from build123d import *

# Parameters (mm, degrees)
ESQUISSE1_W                          = 61
ESQUISSE1_H                          = 41
BOSS_EXTRU_1_DEPTH                   = 100
ENL_V_MAT_EXTRU_1_DEPTH              = 57
ESQUISSE6_W                          = 58
ESQUISSE6_H                          = 3
BOSS_EXTRU_2_DEPTH                   = 4
ESQUISSE7_W                          = 35
ESQUISSE7_H                          = 3
BOSS_EXTRU_3_DEPTH                   = 6
ESQUISSE11_W                         = 58
ESQUISSE11_H                         = 3
BOSS_EXTRU_4_DEPTH                   = 7
ESQUISSE12_W                         = 59.546555331
ESQUISSE12_H                         = 3
BOSS_EXTRU_5_DEPTH                   = 5
R_P_TITION_LIN_AIRE1_COUNT           = 2
R_P_TITION_LIN_AIRE1_PITCH           = 13
R_P_TITION_LIN_AIRE1_COPY_1_SKETCH_W = 59.546555331
R_P_TITION_LIN_AIRE1_COPY_1_SKETCH_H = 3
R_P_TITION_LIN_AIRE1_COPY_1_DEPTH    = 5
ESQUISSE13_W                         = 15
ESQUISSE13_H                         = 3
BOSS_EXTRU_6_DEPTH                   = 5
R_P_TITION_LIN_AIRE3_COUNT           = 2
R_P_TITION_LIN_AIRE3_PITCH           = 4
ESQUISSE14_W                         = 15
ESQUISSE14_H                         = 7
BOSS_EXTRU_7_DEPTH                   = 16
ESQUISSE15_W                         = 2
ESQUISSE15_H                         = 1
ENL_V_MAT_EXTRU_2_DEPTH              = 14
ENL_V_MAT_EXTRU_3_DEPTH              = 15
ESQUISSE17_W                         = 59.954419869
ESQUISSE17_H                         = 3
BOSS_EXTRU_8_DEPTH                   = 15
ESQUISSE18_W                         = 20.5
ESQUISSE18_H                         = 21
ENL_V_MAT_EXTRU_4_DEPTH              = 62


with BuildPart() as part:
    # Esquisse1 → Boss.-Extru.1 (new body)
    with BuildSketch(Plane(origin=(0, 0, 0), x_dir=(1, 0, 0), z_dir=(0, 1, 0))):
        Rectangle(ESQUISSE1_W, ESQUISSE1_H)
    extrude(amount=BOSS_EXTRU_1_DEPTH)

    # Esquisse3 → Enlèv. mat.-Extru.1 (cut)
    with BuildSketch(Plane(origin=(30.5, 0, 0), x_dir=(0, 0, -1), z_dir=(1, 0, 0))):
        Polygon((17.5, 13), (17.5, 97), (-17.5, 97), (-17.5, 3), (14, 3), (14, 13), align=None)
    extrude(amount=-ENL_V_MAT_EXTRU_1_DEPTH, mode=Mode.SUBTRACT)

    # Esquisse6 → Boss.-Extru.2 (add)
    with BuildSketch(Plane(origin=(0, 0, -20.5), x_dir=(-1, 0, 0), z_dir=(0, 0, -1))):
        with Locations((-1.5, 11.5)):
            Rectangle(ESQUISSE6_W, ESQUISSE6_H)
    boss_extru_2 = extrude(amount=-BOSS_EXTRU_2_DEPTH)

    # Symétrie1: Boss.-Extru.2 across plane
    add(boss_extru_2.mirror(Plane.XY))

    # Esquisse7 → Boss.-Extru.3 (add)
    with BuildSketch(Plane.ZY.offset(30.5)):
        with Locations((0, 11.5)):
            Rectangle(ESQUISSE7_W, ESQUISSE7_H)
    extrude(amount=-BOSS_EXTRU_3_DEPTH)

    # Esquisse11 → Boss.-Extru.4 (add)
    with BuildSketch(Plane(origin=(0, 0, -20.5), x_dir=(-1, 0, 0), z_dir=(0, 0, -1))):
        with Locations((-1.5, 11.5)):
            Rectangle(ESQUISSE11_W, ESQUISSE11_H)
    extrude(amount=-BOSS_EXTRU_4_DEPTH)

    # Esquisse12 → Boss.-Extru.5 (add)
    with BuildSketch(Plane(origin=(0, 0, -20.5), x_dir=(-1, 0, 0), z_dir=(0, 0, -1))):
        with Locations((-0.726722335, 51.5)):
            Rectangle(ESQUISSE12_W, ESQUISSE12_H)
    boss_extru_5 = extrude(amount=-BOSS_EXTRU_5_DEPTH)

    # Symétrie2: Boss.-Extru.5 across plane
    add(boss_extru_5.mirror(Plane.XY))

    # Répétition linéaire1: Boss.-Extru.5 ×2
    with Locations(*[(0, -i * R_P_TITION_LIN_AIRE1_PITCH, 0) for i in range(1, R_P_TITION_LIN_AIRE1_COUNT)]):
        add(boss_extru_5)

    # Répétition linéaire1 copy 1 sketch → Répétition linéaire1 copy 1 (add)
    with BuildSketch(Plane(origin=(0, -13, 20.5), x_dir=(-1, 0, 0), z_dir=(0, 0, 1))):
        with Locations((-0.726722335, -51.5)):
            Rectangle(R_P_TITION_LIN_AIRE1_COPY_1_SKETCH_W, R_P_TITION_LIN_AIRE1_COPY_1_SKETCH_H)
    extrude(amount=-R_P_TITION_LIN_AIRE1_COPY_1_DEPTH)

    # Esquisse13 → Boss.-Extru.6 (add)
    with BuildSketch(Plane.XY.offset(20.5)):
        with Locations((-20, 81.5)):
            Rectangle(ESQUISSE13_W, ESQUISSE13_H)
    boss_extru_6 = extrude(amount=-BOSS_EXTRU_6_DEPTH)

    # Répétition linéaire3: Boss.-Extru.6 ×2
    with Locations(*[(0, i * R_P_TITION_LIN_AIRE3_PITCH, 0) for i in range(1, R_P_TITION_LIN_AIRE3_COUNT)]):
        add(boss_extru_6)

    # Esquisse14 → Boss.-Extru.7 (add)
    with BuildSketch(Plane(origin=(0, 0, -20.5), x_dir=(-1, 0, 0), z_dir=(0, 0, -1))):
        with Locations((20, 83.5)):
            Rectangle(ESQUISSE14_W, ESQUISSE14_H)
    extrude(amount=-BOSS_EXTRU_7_DEPTH)

    # Esquisse15 → Enlèv. mat.-Extru.2 (cut)
    with BuildSketch(Plane(origin=(-12.5, 0, 0), x_dir=(0, 0, -1), z_dir=(1, 0, 0))):
        with Locations((4.5, 83.5)):
            Rectangle(ESQUISSE15_W, ESQUISSE15_H)
    extrude(amount=-ENL_V_MAT_EXTRU_2_DEPTH, mode=Mode.SUBTRACT)

    # Esquisse16 → Enlèv. mat.-Extru.3 (cut)
    with BuildSketch(Plane(origin=(0, 100, 0), x_dir=(1, 0, 0), z_dir=(0, 1, 0))):
        with BuildLine():
            Line((15.5, 2), (30.5, 2))
            Line((30.5, 2), (30.5, 17))
            Line((30.5, 17), (15.5, 17))
            ThreePointArc((15.5, 17), (8, 9.5), (15.5, 2))
        make_face()
    extrude(amount=-ENL_V_MAT_EXTRU_3_DEPTH, mode=Mode.SUBTRACT)

    # Esquisse17 → Boss.-Extru.8 (add)
    with BuildSketch(Plane(origin=(0, 0, -20.5), x_dir=(-1, 0, 0), z_dir=(0, 0, -1))):
        with Locations((-0.522790066, 75.5)):
            Rectangle(ESQUISSE17_W, ESQUISSE17_H)
    extrude(amount=-BOSS_EXTRU_8_DEPTH)

    # Esquisse18 → Enlèv. mat.-Extru.4 (cut, through all)
    with BuildSketch(Plane(origin=(30.5, 0, 0), x_dir=(0, 0, -1), z_dir=(1, 0, 0))):
        with Locations((-10.25, 63.5)):
            Rectangle(ESQUISSE18_W, ESQUISSE18_H)
    extrude(amount=-ENL_V_MAT_EXTRU_4_DEPTH, mode=Mode.SUBTRACT)


solid = part.part
The listing builds one solid part. Answer for the finished solid, in the listing's coordinates (mm). A direction names the side the tool comes from. Give positions to 0.01 mm unless a question says otherwise; leave off trailing zeros. Write each loop counter-clockwise with the first axis right and the second up, starting at its lowest first coordinate (ties: lowest second). Pieces come first, ordered by that corner, then holes. Notation, with made-up numbers: (-26.5, 54.25) - (-16.5, 54.25) arc R24 ccw to (-16.5, 76.25) - close; hole circle Ø8 at (88, -14.75). An arc over 180 degrees is marked (long way). Use a Markdown table: item, result.
1. For a pull along Y with two mould halves and no side action, classify faces 1 (the flat face through (-12.5, 85, 17)), 2 (the flat face through (0, 100, 0)), 3 (the flat face through (30.5, 91, 18)) as released by +Y, released by -Y, zero draft, split by the parting line, or undercut.
Values follow:
| item | result |
|---|---|
| face 1 | undercut |
| face 2 | released by +Y |
| face 3 | zero draft |
2. Each of these flat-tipped pins is pushed along its axis until it touches: P1, Ø7.5, axis at y = 8, z = -0.5, coming from the +X side; P2, Ø5, axis at y = 88, z = -9.5, coming from the +X side; P3, Ø8, axis at x = 23, z = -11.5, coming from the +Y side. Where does it stop, or does it pass through?
Values follow:
| item | result |
|---|---|
| P1 | stops at x = -24.5 |
| P2 | stops at x = -12.5 |
| P3 | stops at y = 77 |
3. Section C-C on z = -9.5 is taken. Write down the section's boundary in (x, y).
Values follow:
| item | result |
|---|---|
| outline | (-30.5, 0) - (30.5, 0) - (30.5, 3) - (-26.5, 3) - (-26.5, 10) - (-24.5, 10) - (-24.5, 13) - (-26.5, 13) - (-26.5, 74) - (30.5, 74) - (30.5, 77) - (-26.5, 77) - (-26.5, 80) - (-12.5, 80) - (-12.5, 87) - (-26.5, 87) - (-26.5, 97) - (8, 97) - (8, 100) - (-30.5, 100) - close |
4. Section A-A on z = 11 is taken. Write down the section's boundary in (x, y), plus the area to 3 significant figures.
Values follow:
| item | result |
|---|---|
| outline | (-30.5, 0) - (30.5, 0) - (30.5, 3) - (-26.5, 3) - (-26.5, 10) - (-24.5, 10) - (-24.5, 13) - (-26.5, 13) - (-26.5, 53) - (-30.5, 53) - close; (-30.5, 74) - (-26.5, 74) - (-26.5, 97) - (30.5, 97) - (30.5, 100) - (-30.5, 100) - close |
| area | 664 mm² |
5. A tool of negligible diameter and unlimited length cuts with its end or side. For faces 4 (the flat face through (-7, 74, 18)), 5 (the flat face through (-19, 82, -4.5)), 6 (the flat face through (2, 74, -12)), from which of +Z, -Z, +X, -X, +Y, -Y can it reach the whole face along a straight path? Write none if from no direction.
Values follow:
| item | result |
|---|---|
| face 4 | +Z, +X, -X |
| face 5 | +X |
| face 6 | +Z, +X |
6. Section B-B on y = 20 is taken. Write down the section's boundary in (x, z), plus the area to 3 significant figures.
Values follow:
| item | result |
|---|---|
| outline | (-30.5, -20.5) - (30.5, -20.5) - (30.5, -17.5) - (-26.5, -17.5) - (-26.5, 17.5) - (30.5, 17.5) - (30.5, 20.5) - (-30.5, 20.5) - close |
| area | 506 mm² |
7. Find the intervals of material crossed by probe 1 along Y at (x, z) = (-9.5, -12.5); probe 2 along Y at (x, z) = (-10.5, 17); probe 3 along Y at (x, z) = (25.5, -9), in increasing order. Write a range as from..to.
Values follow:
| item | result |
|---|---|
| probe 1 | y = 0..3, 74..77, 97..100 |
| probe 2 | y = 0..3, 10..13, 37..40, 50..53, 97..100 |
| probe 3 | y = 0..3, 74..77 |
